For this review, take the finished solid that the model builds, in its own axes (mm). Round coordinates to 2 decimals unless told otherwise and drop trailing zeros. Order: outer loops, then holes, each group sorted by start corner. A loop starts at its lowest first (then second) coordinate and runs counter-clockwise, first axis right, second up. Notation, with made-up numbers: (29.5, 70) - (53.5, 70) arc R13 cw to (53.5, 74) - close; hole circle Ø9 at (34, 63). An arc over 180 degrees is marked (long way). One line per item, written item: value.
```python
from build123d import *

# Parameters (mm, degrees)
F1_DEPTH = 17.5
F2_R     = 0.5


with BuildPart() as f1:
    # F0 (on Front) → F1 (new body, symmetric)
    with BuildSketch(Plane.XZ):
        Polygon((-65.75, 1.5), (-65.75, 0), (65.75, 0), (65.75, 1.5), (63.75, 1.5), (-63.75, 1.5), align=None)
        Polygon((-65.75, 3.5), (-65.75, 1.5), (-63.75, 1.5), align=None)
        Polygon((63.75, 1.5), (65.75, 1.5), (65.75, 3.5), align=None)
    extrude(amount=F1_DEPTH, both=True)

    # F2
    f2_edges = [f1.edges().sort_by_distance(p)[0] for p in [
        (-65.75, 0, 3.5),
        (65.75, 0, 3.5),
    ]]
    fillet(f2_edges, radius=F2_R)


solid = f1.part
```
Item 1: The part is to be moulded in two halves that separate along X. For faces 1 (the flat face through (-1, 0, 0)), 2 (the flat face through (65.75, 0, 1)), 3 (the flat face through (1, 0, 1.5)), say which applies: +X half, -X half, draft (parallel to the pull), parting line (faces both ways), or undercut.
Returned:
face 1: draft
face 2: +X half
face 3: undercut
Item 2: Take a section at B-B (x = 36). Write out the cut boundary in (y, z), plus the area to 3 significant figures.
Returned:
outline: (-17.5, 0) - (17.5, 0) - (17.5, 1.5) - (-17.5, 1.5) - close
area: 52.5 mm^2
Item 3: For P1, Ø17.5, axis at x = -13.5, y = -8, coming from the +Z side, flat-tipped, find the tip position at first contact; note if it passes through.
Returned:
P1: z = 1.5
Item 4: Wall thickness on line 1 (Z direction, x = 14, y = -8); line 2 (X direction, y = -4, z = 2.3); line 3 (X direction, y = -8, z = 2.4): over which ranges is each line inside the solid? List them lowest first.
Returned:
line 1: 0 to 1.5
line 2: -65.75 to -64.55, 64.55 to 65.75
line 3: -65.74 to -64.65, 64.65 to 65.74
Item 5: Take a section at A-A (y = -12.5). Write out the cut boundary in (x, z).
Returned:
outline: (-65.75, 0) - (65.75, 0) - (65.75, 2.29) arc R0.5 ccw to (64.9, 2.65) - (63.75, 1.5) - (-63.75, 1.5) - (-64.9, 2.65) arc R0.5 ccw to (-65.75, 2.29) - close
